from build123d import *

# Parameters (mm, degrees)
SKETCH_R        = 70
PAD_DEPTH       = 5
SKETCH001_R     = 4
POCKET_DEPTH    = 5
SKETCH002_R     = 4
POCKET001_DEPTH = 5


with BuildPart() as part:
    # Sketch → Pad (new body)
    with BuildSketch(Plane.XY):
        Circle(SKETCH_R)
    extrude(amount=PAD_DEPTH)

    # Sketch001 → Pocket (cut)
    with BuildSketch(Plane.XY.offset(5)):
        with Locations((-42.426407, 42.426407)):
            Circle(SKETCH001_R)
        with Locations((42.426407, 42.426407)):
            Circle(SKETCH001_R)
        with Locations((42.426407, -42.426407)):
            Circle(SKETCH001_R)
        with Locations((-42.426407, -42.426407)):
            Circle(SKETCH001_R)
    extrude(amount=-POCKET_DEPTH, mode=Mode.SUBTRACT)

    # Sketch002 → Pocket001 (cut)
    with BuildSketch(Plane.XY.offset(5)):
        with Locations((-31, 0)):
            Circle(SKETCH002_R)
        with Locations((31, 0)):
            Circle(SKETCH002_R)
    extrude(amount=-POCKET001_DEPTH, mode=Mode.SUBTRACT)


solid = part.part
Read the model definition and answer for the solid it produces. Units are mm, in the model's axes. Give positions to 0.01 mm unless a question says otherwise; leave off trailing zeros. Write each loop counter-clockwise with the first axis right and the second up, starting at its lowest first coordinate (ties: lowest second). Pieces come first, ordered by that corner, then holes. Notation, with made-up numbers: (39, -17) -> (64, -17) arc R15 ccw to (64, 2) -> close; hole circle Ø3 at (23, -10). An arc over 180 degrees is marked (long way). Answer as a JSON object with one key per item and string values. Group by question number.
1) Each of these flat-tipped pins is pushed along its axis until it touches: P1, Ø7, axis at x = -31, y = 0, coming from the +Z side; P2, Ø1, axis at y = -8, z = 3, coming from the -X side; P3, Ø9, axis at x = 31, y = 0, coming from the -Z side; P4, Ø2, axis at x = 13, z = 1.5, coming from the -Y side. Where does it stop, or does it pass through?
2) Find section D-D (y = 52.5). Write down the section's boundary in (x, z), and give its area (3 significant figures).
3) Find section A-A (y = 0). Write down the section's boundary in (x, z), and give its area (3 significant figures).
4) Find section B-B (x = 31). Write down the section's boundary in (y, z).
5) Consider L1, parallel to X at y = 0.5, z = 2.95; L2, parallel to X at y = 45.5, z = 4.1; L3, parallel to Y at x = 39, z = 0.65. Determine where each line is inside the solid, lowest interval first. Write a range as from..to.
6) The mould has two halves that part along X. Classify faces 1 (the flat face through (-1, 1, 0)), 2 (the cylindrical face through (-55.55, -42.594, 2.465)), 3 (the cylindrical face through (-34.2, -2.4, 2.5)): +X half, -X half, draft (parallel to the pull), parting line (faces both ways), or undercut.
7) Find section C-C (z = 2.25). Write down the section's boundary in (x, y), and give its area (3 significant figures).
Values follow:
{
 "1": {"P1": "passes through", "P2": "stops at x = -69.6", "P3": "stops at z = 0", "P4": "stops at y = -68.96"},
 "2": {"outline": "(-46.3, 0) -> (46.3, 0) -> (46.3, 5) -> (-46.3, 5) -> close", "area": "463 mm2"},
 "3": {"outline": "(-70, 0) -> (-35, 0) -> (-35, 5) -> (-70, 5) -> close; (-27, 0) -> (27, 0) -> (27, 5) -> (-27, 5) -> close; (35, 0) -> (70, 0) -> (70, 5) -> (35, 5) -> close", "area": "620 mm2"},
 "4": {"outline": "(-62.76, 0) -> (-4, 0) -> (-4, 5) -> (-62.76, 5) -> close; (4, 0) -> (62.76, 0) -> (62.76, 5) -> (4, 5) -> close"},
 "5": {"L1": "x = -70..-34.97, -27.03..27.03, 34.97..70", "L2": "x = -53.2..-44.99, -39.87..39.87, 44.99..53.2", "L3": "y = -58.13..-44.49, -40.36..40.36, 44.49..58.13"},
 "6": {"face 1": "draft", "face 2": "parting line", "face 3": "undercut"},
 "7": {"outline": "circle Ø140 at (0, 0); hole circle Ø8 at (-42.43, -42.43); hole circle Ø8 at (-42.43, 42.43); hole circle Ø8 at (-31, 0); hole circle Ø8 at (31, 0); hole circle Ø8 at (42.43, -42.43); hole circle Ø8 at (42.43, 42.43)", "area": "15,100 mm2"}
}
